Read the model definition and answer for the solid it produces. Units are mm, in the model's axes. Face numbers are marked on the shaded views. Give positions to 0.01 mm unless a question says otherwise; leave off trailing zeros. Order: outer loops, then holes, each group sorted by start corner. A loop starts at its lowest first (then second) coordinate and runs counter-clockwise, first axis right, second up.
```python
from build123d import *

# Parameters (mm, degrees)
SKETCH1_W           = 38.1
SKETCH1_H           = 101.6
SKETCH1_R           = 10.7061
BOSS_EXTRUDE1_DEPTH = 6.35
CUT_EXTRUDE1_REACH  = 110.694
SKETCH2_R           = 4.445
FILLET1_R           = 5


with BuildPart() as part:
    # Sketch1 → Boss-Extrude1 (new body)
    with BuildSketch(Plane.XY):
        with Locations((19.05, -50.8)):
            Rectangle(SKETCH1_W, SKETCH1_H)
        with Locations((17.272, -61.6)):
            Circle(SKETCH1_R, mode=Mode.SUBTRACT)
    extrude(amount=BOSS_EXTRUDE1_DEPTH)

    # Sketch2 → Cut-Extrude1 (cut, up to next)
    with BuildSketch(Plane.XY.offset(6.35), mode=Mode.PRIVATE) as cut_extrude1_sk1:
        with Locations((19.05, -23.588381621)):
            Circle(SKETCH2_R)
    cut_extrude1_tool1 = extrude(cut_extrude1_sk1.sketch, amount=-CUT_EXTRUDE1_REACH, mode=Mode.PRIVATE) & part.part
    # Sketch2 → Cut-Extrude1 (cut, up to next)
    with BuildSketch(Plane.XY.offset(6.35), mode=Mode.PRIVATE) as cut_extrude1_sk2:
        with Locations((19.05, -86.425541616)):
            Circle(SKETCH2_R)
    cut_extrude1_tool2 = extrude(cut_extrude1_sk2.sketch, amount=-CUT_EXTRUDE1_REACH, mode=Mode.PRIVATE) & part.part
    add(cut_extrude1_tool1.solids().sort_by_distance((19.05, -23.588382, 6.35))[0], mode=Mode.SUBTRACT)
    add(cut_extrude1_tool2.solids().sort_by_distance((19.05, -86.425542, 6.35))[0], mode=Mode.SUBTRACT)

    # Fillet1
    fillet1_edges = [part.edges().sort_by_distance(p)[0] for p in [
        (0, 0, 3.175),
        (38.1, 0, 3.175),
        (38.1, -101.6, 3.175),
        (0, -101.6, 3.175),
    ]]
    fillet(fillet1_edges, radius=FILLET1_R)


solid = part.part
```
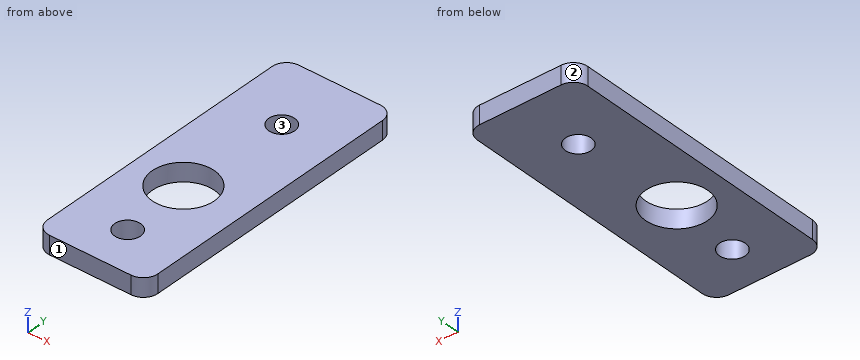
1) The part is cut by section B-B on x = 9. Determine the outline of the cut face in (y, z), and give its area (3 significant figures).
Final values:
outline: (-101.6, 0) - (-68.4, 0) - (-68.4, 6.35) - (-101.6, 6.35) - close; (-54.8, 0) - (0, 0) - (0, 6.35) - (-54.8, 6.35) - close
area: 559 mm2
2) The part is cut by section A-A on y = -61.6. Determine the outline of the cut face in (x, z).
Final values:
outline: (0, 0) - (6.57, 0) - (6.57, 6.35) - (0, 6.35) - close; (27.98, 0) - (38.1, 0) - (38.1, 6.35) - (27.98, 6.35) - close
3) Consider L1, parallel to X at y = -86, z = 1.5; L2, parallel to Y at x = 19.05, z = 4.25; L3, parallel to Y at x = 18.5, z = 1. Determine where each line is inside the solid, lowest interval first.
Final values:
L1: x = 0 to 14.63, 23.47 to 38.1
L2: y = -101.6 to -90.87, -81.98 to -72.16, -51.04 to -28.03, -19.14 to 0
L3: y = -101.6 to -90.84, -82.01 to -72.24, -50.96 to -28, -19.18 to 0
4) For a pull along X with two mould halves and no side action, classify the marked faces 1, 2 and 3 as released by +X, released by -X, zero draft, split by the parting line, or undercut.
Final values:
face 1: zero draft
face 2: released by -X
face 3: undercut
5) The part is cut by section C-C on x = 19.05. Determine the outline of the cut face in (y, z).
Final values:
outline: (-101.6, 0) - (-90.87, 0) - (-90.87, 6.35) - (-101.6, 6.35) - close; (-81.98, 0) - (-72.16, 0) - (-72.16, 6.35) - (-81.98, 6.35) - close; (-51.04, 0) - (-28.03, 0) - (-28.03, 6.35) - (-51.04, 6.35) - close; (-19.14, 0) - (0, 0) - (0, 6.35) - (-19.14, 6.35) - close
6) The part is cut by section D-D on z = 1. Determine the outline of the cut face in (x, y) (3 decimals).
Final values:
outline: (0, -96.6) arc R5 ccw to (5, -101.6) - (33.1, -101.6) arc R5 ccw to (38.1, -96.6) - (38.1, -5) arc R5 ccw to (33.1, 0) - (5, 0) arc R5 ccw to (0, -5) - close; hole circle Ø21.412 at (17.272, -61.6); hole circle Ø8.89 at (19.05, -86.426); hole circle Ø8.89 at (19.05, -23.588)
7) Given pin 1 (17 mm diameter, centred on x = 17.272, y = -61.6, fed in from +Z), flat-ended and moving along its own axis, determine where the tip first touches the part or whether it passes through.
Final values:
pin 1: passes through
